Read the model definition and answer for the solid it produces. Units are mm, in the model's axes. Face numbers are marked on the shaded views. Give positions to 0.01 mm unless a question says otherwise; leave off trailing zeros. Order: outer loops, then holes, each group sorted by start corner. A loop starts at its lowest first (then second) coordinate and runs counter-clockwise, first axis right, second up.
```python
from build123d import *

# Parameters (mm, degrees)
ESBO_O1_R                                            = 1.6
RESSALTO_EXTRUS_O1_DEPTH                             = 30
ESCAREADO_PARA_PARAFUSO_DE_M_QUINA_COM_C_D           = 3.4544
ESCAREADO_PARA_PARAFUSO_DE_M_QUINA_COM_C_CSINK_D     = 6.4008
ESCAREADO_PARA_PARAFUSO_DE_M_QUINA_COM_C_CSINK_ANGLE = 82
CORTE_EXTRUS_O3_DEPTH                                = 10
ESBO_O28_R                                           = 2.758385
CORTE_EXTRUS_O8_DEPTH                                = 10


with BuildPart() as part:
    # Esboço1 → Ressalto-extrusão1 (new body)
    with BuildSketch(Plane.XY):
        with BuildLine():
            Line((0, -10), (0, -21.90721))
            ThreePointArc((0, -21.90721), (2.928932, -28.978277), (10, -31.90721))
            Line((10, -31.90721), (28.375876, -31.90721))
            ThreePointArc((28.375876, -31.90721), (35.446943, -28.978277), (38.375876, -21.90721))
            Line((38.375876, -21.90721), (38.375876, -10))
            ThreePointArc((38.375876, -10), (35.446943, -2.928932), (28.375876, 0))
            Line((28.375876, 0), (10, 0))
            ThreePointArc((10, 0), (2.928932, -2.928932), (0, -10))
        make_face()
        with Locations((28.375876, -10)):
            Circle(ESBO_O1_R, mode=Mode.SUBTRACT)
        with Locations((10, -10)):
            Circle(ESBO_O1_R, mode=Mode.SUBTRACT)
        with Locations((10, -21.90721)):
            Circle(ESBO_O1_R, mode=Mode.SUBTRACT)
        with Locations((28.375876, -21.90721)):
            Circle(ESBO_O1_R, mode=Mode.SUBTRACT)
    extrude(amount=RESSALTO_EXTRUS_O1_DEPTH)

    # Escareado para parafuso de máquina com cabeça oval de #52 (through all)
    with Locations(Plane.XY.offset(30)):
        with Locations((10, -10), (28.375876, -10), (28.375876, -21.90721), (10, -21.90721)):
            CounterSinkHole(ESCAREADO_PARA_PARAFUSO_DE_M_QUINA_COM_C_D / 2, ESCAREADO_PARA_PARAFUSO_DE_M_QUINA_COM_C_CSINK_D / 2, counter_sink_angle=ESCAREADO_PARA_PARAFUSO_DE_M_QUINA_COM_C_CSINK_ANGLE)

    # Esboço23 → Corte-extrusão3 (cut)
    with BuildSketch(Plane(origin=(0, 0, 0), x_dir=(-1, 0, 0), z_dir=(0, 0, -1))):
        Polygon((-19.187938, -15.953605), (-28.375876, -10), (-28.375876, -21.90721), align=None)
        with BuildLine():
            ThreePointArc((-19.183742, -15.950886), (-19.182938, -15.953605), (-19.183742, -15.956324))
            Line((-19.183742, -15.956324), (-10, -21.90721))
            Line((-10, -21.90721), (-10, -10))
            Line((-10, -10), (-19.183742, -15.950886))
        make_face()
    extrude(amount=-CORTE_EXTRUS_O3_DEPTH, mode=Mode.SUBTRACT)

    # Esboço28 → Corte-extrusão8 (cut)
    with BuildSketch(Plane(origin=(0, 0, 0), x_dir=(-1, 0, 0), z_dir=(0, 0, -1))):
        with Locations((-19.183742, -15.956324)):
            Circle(ESBO_O28_R)
    extrude(amount=-CORTE_EXTRUS_O8_DEPTH, mode=Mode.SUBTRACT)

    # Esboço29 → bola (revolve)
    with BuildSketch(Plane.XY.offset(30)):
        with BuildLine():
            ThreePointArc((21.285981, -14.594114), (17.828447, -13.855562), (17.089895, -17.313096))
            Line((17.089895, -17.313096), (21.285981, -14.594114))
        make_face()
        with BuildLine():
            Line((21.285981, -14.594114), (17.089895, -17.313096))
            ThreePointArc((17.089895, -17.313096), (19.896772, -18.35101), (21.687938, -15.953605))
            ThreePointArc((21.687938, -15.953605), (21.585343, -15.24477), (21.285981, -14.594114))
        make_face()
    revolve(axis=Axis((10, -21.90721, 30), (0.8392171833395659, 0.5437963949748155, 0)))


solid = part.part
```
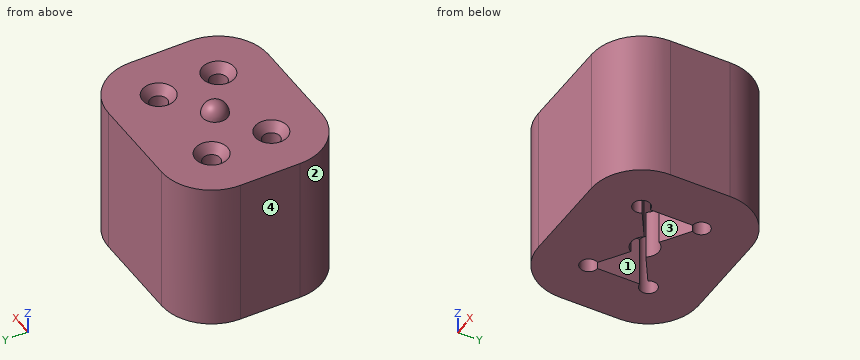
1) The part is cut by section C-C on y = -3.5. Determine the outline of the cut face in (x, z), and give its area (3 significant figures).
Final values:
outline: (2.4, 0) - (35.98, 0) - (35.98, 30) - (2.4, 30) - close
area: 1,010 mm2
2) The part is cut by section D-D on x = 16. Determine the outline of the cut face in (y, z), and give its area (3 significant figures).
Final values:
outline: (-31.91, 0) - (-18.02, 0) - (-18.02, 10) - (-13.89, 10) - (-13.89, 0) - (0, 0) - (0, 30) - (-31.91, 30) - close
area: 916 mm2
3) The part is cut by section A-A on x = 24. Determine the outline of the cut face in (y, z).
Final values:
outline: (-31.91, 0) - (-19.07, 0) - (-19.07, 10) - (-12.84, 10) - (-12.84, 0) - (0, 0) - (0, 30) - (-31.91, 30) - close
4) For a pull along Y with two mould halves and no side action, classify the marked faces 1, 2, 3 and 4 as released by +Y, released by -Y, zero draft, split by the parting line, or undercut.
Final values:
face 1: undercut
face 2: released by -Y
face 3: undercut
face 4: zero draft
5) Given pin 1 (6 mm diameter, centred on x = 23, y = -9.5, fed in from -Z); pin 2 (16 mm diameter, centred on x = 27, y = -12.5, fed in from +Z); pin 3 (1 mm diameter, centred on x = 25.5, y = -6.5, fed in from +Z); pin 4 (2 mm diameter, centred on x = 10, y = -10, fed in from -Z), each flat-ended and moving along its own axis, determine where each tip first touches the part or whether it passes through.
Final values:
pin 1: stops at z = 0
pin 2: stops at z = 32.44
pin 3: stops at z = 30
pin 4: passes through
6) The part is cut by section B-B on x = 10.5. Count the separate pieces of the cut face and the enclosed holes in it, and give its area (3 significant figures).
Final values:
separate pieces: 3
enclosed holes: 0
area: 668 mm2
7) Consider L1, parallel to X at y = -10, z = 4; L2, parallel to Y at x = 10, z = 17; L3, parallel to Y at x = 27.5, z = 22. Determine where each line is inside the solid, lowest interval first.
Final values:
L1: x = 0 to 8.27, 11.73 to 26.65, 30.1 to 38.38
L2: y = -31.91 to -23.63, -20.18 to -11.73, -8.27 to 0
L3: y = -31.91 to -23.4, -20.42 to -11.49, -8.51 to 0
